Could you check a few things on this model? Use its own coordinates, in mm. Face numbers are marked on the shaded views. A direction names the side the tool comes from. Give positions to 0.01 mm unless a question says otherwise; leave off trailing zeros. Order: outer loops, then holes, each group sorted by start corner. A loop starts at its lowest first (then second) coordinate and runs counter-clockwise, first axis right, second up. Notation, with made-up numbers: M 57.5,67 L 79.5,67 A7 cw 79.5,72 Z; hole C 68,-28 d3. An arc over 180 degrees is marked long. Use a Markdown table: item, result. Add a question column.
Item 1: Suppose I cut it at B-B on x = -3. Write out the boundary of the cut face in (y, z).
Item 2: I'm going to push flat-ended pins straight in: pin 1 Ø3 at (x, y) = (-11.5, -11.5) entering from -Z; pin 2 Ø6 at (x, z) = (-12.5, -12.5) entering from +Y. Where does each tip first touch, or does it pass through?
Item 3: If I drill on L1, parallel to X at y = -12.5, z = -20; L2, parallel to Y at x = 12.5, z = -18; L3, parallel to Y at x = 12, z = 17, over which ranges is the centre line in solid material (lowest first)? Write a range as from..to.
Item 4: If we mould it in two halves opening along X, with no side actions, what happens to the marked faces 1, 2 and 3? For each: released by +X, released by -X, zero draft, split by the parting line, or undercut.
Item 5: For the marked faces 4, 5 and 6, which set-ups out of +Z, -Z, +X, -X, +Y, -Y let a thin tool reach every point of the face, with its end or its side?
Item 6: Suppose I cut it at D-D on x = 21. Write out the boundary of the cut face in (y, z), plus the area to 3 significant figures.
from build123d import *

# Parameters (mm, degrees)
F0_W      = 50
F0_H      = 50
F1_DEPTH  = 50
F2_R      = 5
F3_DEPTH  = 10
F6_R      = 5
F7_DEPTH  = 10
F5_R      = 5
F8_DEPTH  = 5
F9_R      = 5
F10_DEPTH = 10
F11_R     = 5
F12_DEPTH = 10
F13_R     = 5
F14_DEPTH = 10
F15_R     = 5


with BuildPart() as f1:
    # F0 (on Front) → F1 (new body)
    with BuildSketch(Plane.XZ):
        Rectangle(F0_W, F0_H)
    extrude(amount=F1_DEPTH)

    # F2 (on face) → F3 (cut)
    with BuildSketch(Plane.XZ.offset(50)):
        Circle(F2_R)
    extrude(amount=-F3_DEPTH, mode=Mode.SUBTRACT)

    # F6 (on face) → F7 (cut)
    with BuildSketch(Plane.YZ.offset(25)):
        with Locations((-12.5, 0)):
            Circle(F6_R)
        with Locations((-37.5, 0)):
            Circle(F6_R)
    extrude(amount=-F7_DEPTH, mode=Mode.SUBTRACT)

    # F5 (on face) → F8 (cut)
    with BuildSketch(Plane(origin=(0, 0, 0), x_dir=(-1, 0, 0), z_dir=(0, 1, 0))):
        with Locations((12.5, -12.5)):
            Circle(F5_R)
        with Locations((12.5, 0)):
            Circle(F5_R)
        with Locations((12.5, 12.5)):
            Circle(F5_R)
        with Locations((-12.5, -12.5)):
            Circle(F5_R)
        with Locations((-12.5, 0)):
            Circle(F5_R)
        with Locations((-12.5, 12.5)):
            Circle(F5_R)
    extrude(amount=-F8_DEPTH, mode=Mode.SUBTRACT)

    # F9 (on face) → F10 (cut)
    with BuildSketch(Plane(origin=(-25, 0, 0), x_dir=(0, -1, 0), z_dir=(-1, 0, 0))):
        with Locations((12.5, 0)):
            Circle(F9_R)
        with Locations((37.5, -12.5)):
            Circle(F9_R)
        with Locations((37.5, 12.5)):
            Circle(F9_R)
    extrude(amount=-F10_DEPTH, mode=Mode.SUBTRACT)

    # F11 (on face) → F12 (cut)
    with BuildSketch(Plane.XY.offset(25)):
        with Locations((-12.5, -37.5)):
            Circle(F11_R)
        with Locations((-12.5, -12.5)):
            Circle(F11_R)
        with Locations((12.5, -12.5)):
            Circle(F11_R)
        with Locations((12.5, -37.5)):
            Circle(F11_R)
    extrude(amount=-F12_DEPTH, mode=Mode.SUBTRACT)

    # F13 (on face) → F14 (cut)
    with BuildSketch(Plane(origin=(0, 0, -25), x_dir=(1, 0, 0), z_dir=(0, 0, -1))):
        with Locations((-12.5, 37.5)):
            Circle(F13_R)
        with Locations((12.5, 37.5)):
            Circle(F13_R)
        with Locations((0, 25)):
            Circle(F13_R)
        with Locations((-12.5, 12.5)):
            Circle(F13_R)
        with Locations((12.5, 12.5)):
            Circle(F13_R)
    extrude(amount=-F14_DEPTH, mode=Mode.SUBTRACT)

    # F15
    f15_edges = [f1.edges().sort_by_distance(p)[0] for p in [
        (0, -50, -25),
        (25, -25, -25),
        (25, -50, 0),
        (25, 0, 0),
        (0, 0, -25),
        (-25, -25, -25),
        (-25, -50, 0),
        (-25, 0, 0),
        (0, 0, 25),
        (-25, -25, 25),
        (0, -50, 25),
        (25, -25, 25),
    ]]
    fillet(f15_edges, radius=F15_R)


solid = f1.part
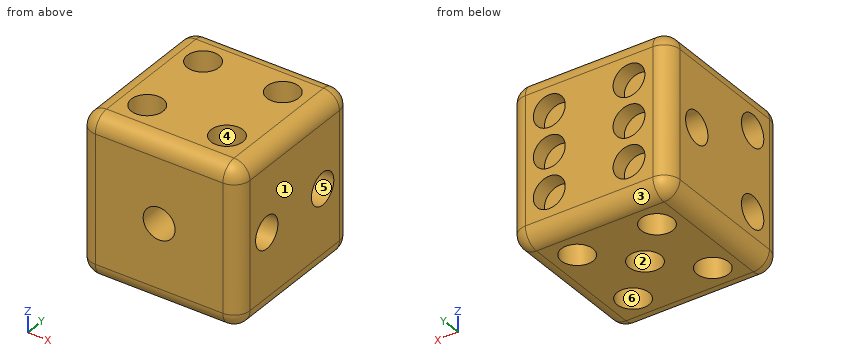
Findings below:
| question | item | result |
|---|---|---|
| 1 | outline | M -50,-20 A5 ccw -45,-25 L -29,-25 L -29,-15 L -21,-15 L -21,-25 L -5,-25 A5 ccw 0,-20 L 0,20 A5 ccw -5,25 L -45,25 A5 ccw -50,20 L -50,4 L -40,4 L -40,-4 L -50,-4 Z |
| 2 | pin 1 | stops at z = -15 |
| 2 | pin 2 | stops at y = -5 |
| 3 | L1 | x = -25..-17.5, -7.5..7.5, 17.5..25 |
| 3 | L2 | y = -50..-42.5, -32.5..-17.5, -7.5..0 |
| 3 | L3 | y = -50..-42.47, -32.53..-17.47, -7.53..-5 |
| 4 | face 1 | released by +X |
| 4 | face 2 | undercut |
| 4 | face 3 | zero draft |
| 5 | face 4 | +Z |
| 5 | face 5 | +X |
| 5 | face 6 | -Z |
| 6 | outline | M -49.9,-20 A4.9 ccw -45,-24.9 L -5,-24.9 A4.9 ccw -0.1,-20 L -0.1,20 A4.9 ccw -5,24.9 L -45,24.9 A4.9 ccw -49.9,20 Z; hole C -37.5,0 d10; hole C -12.5,0 d10 |
| 6 | area | 2,300 mm^2 |
